Verification items for the finished model (mm, model axes). Give positions to 0.01 mm unless a question says otherwise; leave off trailing zeros. Order: outer loops, then holes, each group sorted by start corner. A loop starts at its lowest first (then second) coordinate and runs counter-clockwise, first axis right, second up. Notation, with made-up numbers: (-31, -2) - (3, -2) arc R12 ccw to (3, 7) - close; hole circle Ø7 at (-23.75, -39.75). An arc over 180 degrees is marked (long way). Answer as a JSON object with one key per item and string values.
Autodesk Inventor part; units mm, degrees
ref_plane "YZ Plane" through (0, 0, 0) normal (1, 0, 0) x (0, 1, 0)
ref_plane "XZ Plane" through (0, 0, 0) normal (0, 1, 0) x (-1, 0, 0)
ref_plane "XY Plane" through (0, 0, 0) normal (0, 0, 1) x (1, 0, 0)
sketch "Sketch1" plane through (0, 0, 0) normal (0, 1, 0) x (-1, 0, 0)
  circle A0 centre (28.2679, -64.7457) radius 1.6
  circle A1 centre (-28.2679, -64.7457) radius 1.6
  arc A2 (31.2679, -64.7457) -> (28.2679, -61.7457) centre (28.2679, -64.7457) ccw
  arc A3 (-28.2679, -61.7457) -> (-31.2679, -64.7457) centre (-28.2679, -64.7457) ccw
  line L0 (-28.2679, -61.7457) -> (28.2679, -61.7457)
  line L1 (48.3297, -88.9468) -> (2.1402, -66.9602)
  line L2 (-2.1585, -66.9605) -> (-48.3297, -88.9468)
  arc A4 (2.1402, -66.9602) -> (-2.1585, -66.9605) centre (-0.0088, -71.4748) ccw
  line L3 (-0.0092, -65.9371) -> (-0.0092, -75.9371)
  line L4 (-0.0092, -75.9371) -> (28.2679, -75.9371)
  line L5 (-0.0092, -75.9371) -> (-28.2679, -75.9371)
  line L6 (-31.2679, -72.9371) -> (-31.2679, -64.7457)
  line L7 (31.2679, -64.7457) -> (31.2679, -72.9371)
  arc A5 (28.2679, -75.9371) -> (31.2679, -72.9371) centre (28.2679, -72.9371) ccw
  arc A6 (-31.2679, -72.9371) -> (-28.2679, -75.9371) centre (-28.2679, -72.9371) ccw
  point P0 (0, 0)
  dimension "d0" = 3.2
  dimension "d1" = 3
  dimension "d2" = 3
  dimension "d3" = 5
  dimension "d4" = 10
  dimension "d5" = 3
  dimension "d8" = 14.1913
  dimension "d9" = 62.5358
extrude "Extrusion1" add sketch "Sketch1" along normal blind 1
properties part number "Light sensor ball guard"
(1) Gauge pin test, flat end, axial feed: pin 1 Ø2.5 at (x, z) = (-28.27, -64.75) entering from -Y. Record the tip position at first contact, or that the pin passes through.
Computed values:
{"pin 1": "passes through"}
(2) Section check A-A (y = 0.2). Record the cut outline in (x, z), then the cut area to 3 significant figures.
Computed values:
{"outline": "(-31.27, -72.94) arc R3 ccw to (-28.27, -75.94) - (28.27, -75.94) arc R3 ccw to (31.27, -72.94) - (31.27, -64.75) arc R3 ccw to (28.27, -61.75) - (-28.27, -61.75) arc R3 ccw to (-31.27, -64.75) - close; hole circle Ø3.2 at (-28.27, -64.75); hole circle Ø3.2 at (28.27, -64.75)", "area": "864 mm²"}
(3) Material ranges on line 1 along X through (y, z) = (0.4, -63.75); line 2 along X through (y, z) = (0.25, -62.75); line 3 along Z through (x, y) = (28.5, 0.7), recorded low to high. Write a range as [from, to].
Computed values:
{"line 1": "x = [-31.1, -29.52], [-27.02, 27.02], [29.52, 31.1]", "line 2": "x = [-30.51, 30.51]", "line 3": "z = [-75.93, -66.33], [-63.16, -61.75]"}
(4) Release check for a two-part mould opening along Z. For faces 1 (the cylindrical face through (27.53, 0.493, -63.326)), 2 (the cylindrical face through (-27.921, 0.493, -63.184)), 3 (the flat face through (-31.268, 0.5, -68.8)), 4 (the flat face through (0.4, 0.5, -61.746)) record: pulls with the +Z half, pulls with the -Z half, needs draft (parallel to the pull), parting line crosses it, or undercut.
Computed values:
{"face 1": "undercut", "face 2": "undercut", "face 3": "needs draft", "face 4": "pulls with the +Z half"}
